Verification items for the finished model (mm, model axes). A direction names the side the tool comes from. Round coordinates to 2 decimals unless told otherwise and drop trailing zeros. Write each loop counter-clockwise with the first axis right and the second up, starting at its lowest first coordinate (ties: lowest second). Pieces come first, ordered by that corner, then holes. Notation, with made-up numbers: (6, 26) -> (10, 26) arc R9 cw to (10, 34) -> close; hole circle Ø5 at (53, -23.5). An arc over 180 degrees is marked (long way). Answer as a JSON object with one key per item and string values. Group by question number.
(1) Scan lines: L1, parallel to Z at x = -3.5, y = -3.25; L2, parallel to Y at x = 0, z = 0.6; L3, parallel to Z at x = -1.75, y = 4.75. Record each from-to range of solid material in increasing order. Write a range as from..to.
(2) Draft check along X on faces 1 (the face through (-1.38, -6.2, 0.71)), 2 (the face through (2, -5, 1.372)), 3 (the face through (-3.565, -2.733, 5.368)). Enter one of: released by +X, released by -X, zero draft, split by the parting line, or undercut.
(3) Sectioned sample at C-C on z = 2.25. Record the cut outline in (x, y), and give its area (3 significant figures).
(4) Set-up check for faces 4 (the face through (-1.08, -4.88, 5.63)), 5 (the face through (0, 0, -0.229)), 6 (the face through (0, 0, -0.737)): record each of +Z, -Z, +X, -X, +Y, -Y from which the full face is reachable in a straight line by a thin tool's end or side.
(5) Gauge pin test, flat ends, axial feed: pin 1 Ø2 at (y, z) = (-3.5, 6) entering from -X; pin 2 Ø1 at (x, z) = (-4.5, 4.5) entering from -Y; pin 3 Ø3 at (x, z) = (-4.5, 2.5) entering from +Y. Record the tip position at first contact, or that the pin passes through.
(6) Sectioned sample at A-A on x = 0. Record the cut outline in (y, z), and give its area (3 significant figures).
(7) Sectioned sample at D-D on z = 0.5. Record the cut outline in (x, y).
```python
from build123d import *

# Parameters (mm, degrees)
F0_R          = 5
F1_DEPTH      = 10
F0_R_2        = 6.35
F2_DEPTH      = 1.3716
F2_DEPTH_BACK = 0.7366
F3_T          = -0.508
F4_R          = 0.762


with BuildPart() as f1:
    # F0 (on Top) → F1 (new body)
    with BuildSketch(Plane.XY):
        Circle(F0_R)
    extrude(amount=F1_DEPTH)

    # F0 (on Top) → F2 (join, two sides)
    with BuildSketch(Plane.XY) as f2_sk:
        Circle(F0_R_2)
        Circle(F0_R, mode=Mode.SUBTRACT)
        Circle(F0_R)
    extrude(amount=F2_DEPTH)
    extrude(f2_sk.sketch, amount=-F2_DEPTH_BACK)

    # F3
    f3_openings = [f1.faces().sort_by_distance(p)[0] for p in [
        (0, 0, 10),
    ]]
    offset(amount=F3_T, openings=f3_openings, kind=Kind.INTERSECTION)

    # F4
    f4_edges = [f1.edges().sort_by_distance(p)[0] for p in [
        (-6.35, 0, -0.7366),
    ]]
    fillet(f4_edges, radius=F4_R)


solid = f1.part
```
Computed values:
{
 "1": {"L1": "-0.74..-0.23, 0.86..10", "L2": "-6.35..-5.84, 5.84..6.35", "L3": "-0.74..-0.23, 0.86..1.37"},
 "2": {"face 1": "split by the parting line", "face 2": "zero draft", "face 3": "undercut"},
 "3": {"outline": "circle Ø10 at (0, 0); hole circle Ø8.98 at (0, 0)", "area": "15.1 mm2"},
 "4": {"face 4": "+Z", "face 5": "none", "face 6": "-Z, +X, -X, +Y, -Y"},
 "5": {"pin 1": "x = -4.33", "pin 2": "y = -3", "pin 3": "y = 5.29"},
 "6": {"outline": "(-6.35, 0.03) arc R0.76 ccw to (-5.59, -0.74) -> (5.59, -0.74) arc R0.76 ccw to (6.35, 0.03) -> (6.35, 1.37) -> (5, 1.37) -> (5, 10) -> (4.49, 10) -> (4.49, 0.86) -> (5.84, 0.86) -> (5.84, -0.23) -> (-5.84, -0.23) -> (-5.84, 0.86) -> (-4.49, 0.86) -> (-4.49, 10) -> (-5, 10) -> (-5, 1.37) -> (-6.35, 1.37) -> close", "area": "18.0 mm2"},
 "7": {"outline": "circle Ø12.7 at (0, 0); hole circle Ø11.68 at (0, 0)"}
}
